from build123d import *

# Parameters (mm, degrees)
SKETCH1_R           = 0.6
BOSS_EXTRUDE1_DEPTH = 3
SKETCH1_22_R        = 0.9
SKETCH1_22_R_2      = 0.3
BOSS_EXTRUDE2_DEPTH = 8
SKETCH1_23_R        = 0.8
SKETCH1_23_R_2      = 0.3
BOSS_EXTRUDE3_DEPTH = 5


with BuildPart() as part:
    # Sketch1 → Boss-Extrude1 (new body)
    with BuildSketch(Plane(origin=(0, 0, 0), x_dir=(1, 0, 0), z_dir=(0, 1, 0))):
        with BuildLine():
            ThreePointArc((0.1641009, 1.993256355), (0.024548565, 1.994973575), (-0.113883759, 1.977245221))
            Line((-0.113883759, 1.977245221), (-4.183235691, 1.164159973))
            ThreePointArc((-4.183235691, 1.164159973), (-4.514100231, 1.033532975), (-4.77830642, 0.795352694))
            ThreePointArc((-4.77830642, 0.795352694), (-5.05, 0), (-4.77830642, -0.795352694))
            ThreePointArc((-4.77830642, -0.795352694), (-4.514100231, -1.033532975), (-4.183235691, -1.164159973))
            Line((-4.183235691, -1.164159973), (-0.11388376, -1.977245221))
            ThreePointArc((-0.11388376, -1.977245221), (0.024548564, -1.994973575), (0.164100898, -1.993256355))
            ThreePointArc((0.164100898, -1.993256355), (2, -1e-09), (0.1641009, 1.993256355))
        make_face()
        with Locations(Location((-1.25, 0, 0), (0, 0, 270))):
            Circle(SKETCH1_R, mode=Mode.SUBTRACT)
    extrude(amount=BOSS_EXTRUDE1_DEPTH)

    # Sketch1_22 → Boss-Extrude2 (add)
    # profile 1 of 2: a face of its own
    with BuildSketch(Plane(origin=(0, 0, 0), x_dir=(1, 0, 0), z_dir=(0, 1, 0))):
        with Locations(Location((0.5, 0, 0), (0, 0, 270))):
            Circle(SKETCH1_22_R)
        with Locations((0.5, 0)):
            Circle(SKETCH1_22_R_2, mode=Mode.SUBTRACT)
    # profile 2 of 2: a face of its own
    with BuildSketch(Plane(origin=(0, 0, 0), x_dir=(1, 0, 0), z_dir=(0, 1, 0))):
        with Locations((0.5, 0)):
            Circle(SKETCH1_22_R_2)
    extrude(amount=BOSS_EXTRUDE2_DEPTH)

    # Sketch1_23 → Boss-Extrude3 (add)
    # profile 1 of 2: a face of its own
    with BuildSketch(Plane(origin=(0, 0, 0), x_dir=(1, 0, 0), z_dir=(0, 1, 0))):
        with Locations(Location((-3, 0, 0), (0, 0, 270))):
            Circle(SKETCH1_23_R)
        with Locations((-3, 0)):
            Circle(SKETCH1_23_R_2, mode=Mode.SUBTRACT)
    # profile 2 of 2: a face of its own
    with BuildSketch(Plane(origin=(0, 0, 0), x_dir=(1, 0, 0), z_dir=(0, 1, 0))):
        with Locations((-3, 0)):
            Circle(SKETCH1_23_R_2)
    extrude(amount=BOSS_EXTRUDE3_DEPTH)


solid = part.part
Geometry check sheet. Reference: the model listing, model coordinates, mm. A direction names the side the tool comes from. Give positions to 0.01 mm unless a question says otherwise; leave off trailing zeros. Write each loop counter-clockwise with the first axis right and the second up, starting at its lowest first coordinate (ties: lowest second). Pieces come first, ordered by that corner, then holes. Notation, with made-up numbers: M 10.5,30.25 L 30.5,30.25 A14 ccw 30.5,41.25 Z; hole C -38,28.25 d1. An arc over 180 degrees is marked long. Answer as CSV lines item,"result". Start each with the question number.
Q1. Section check D-D, the plane z = -0.5. Record the cut outline in (x, y).
Q2. Section check C-C, the plane y = 5.5. Record the cut outline in (x, z).
Q3. Tool access check on faces 1 (the face through (-3.78, 3.99, -0.17)), 2 (the face through (-3, 5, 0)), 3 (the face through (-2, 0, 1)). Record the directions out of +Z, -Z, +X, -X, +Y, -Y that give a thin tool (end or side, any length) a straight path to the whole face; none if there is none.
Q4. Section check A-A, the plane z = 0. Record the cut outline in (x, y), then the cut area to 4 significant figures.
Q5. Material ranges on L1, parallel to X at y = 2.25, z = -0.35; L2, parallel to Y at x = -0.5, z = 1.1; L3, parallel to Z at x = 0.5, y = 7.25, recorded low to high.
Q6. Release check for a two-part mould opening along X. For faces 4 (the face through (1.39, 5.46, -0.12)), 5 (the face through (-2.12, 1.479, -1.576)), 6 (the face through (2, 1, 0)), 7 (the face through (1, 8, 0)) record: pulls with the +X half, pulls with the -X half, needs draft (parallel to the pull), parting line crosses it, or undercut.
Q7. Section check B-B, the plane x = -1.25. Record the cut outline in (y, z), then the cut area to 3 significant figures.
Q8. Go/stop test with flat-tipped pins: pin 1 (1.6 mm diameter, centred on x = -1.25, z = 0, fed in from +Y); pin 2 (1.3 mm diameter, centred on x = -3, z = 0.5, fed in from +Y); pin 3 (1 mm diameter, centred on x = -4, y = 4.5, fed in from +Z). Record where each tip stops, or that it passes through.
Geometry says:
1,outline,"M -4.95,0 L -1.58,0 L -1.58,3 L -2.38,3 L -2.38,5 L -3.62,5 L -3.62,3 L -4.95,3 Z; M -0.92,0 L 1.94,0 L 1.94,3 L 1.25,3 L 1.25,8 L -0.25,8 L -0.25,3 L -0.92,3 Z"
2,outline,"C 0.5,0 d1.8"
3,face 1,"+Y"
3,face 2,"+Z, -Z, -X, +Y"
3,face 3,"+Z, -Z, +X, -X, -Y"
4,outline,"M -5.05,0 L -1.85,0 L -1.85,3 L -2.2,3 L -2.2,5 L -3.8,5 L -3.8,3 L -5.05,3 Z; M -0.65,0 L 2,0 L 2,3 L 1.4,3 L 1.4,8 L -0.4,8 L -0.4,3 L -0.65,3 Z"
4,area,"29.75 mm^2"
5,L1,"-5 to -1.74, -0.76 to 1.97"
5,L2,"0 to 3"
5,L3,"-0.9 to 0.9"
6,face 4,"undercut"
6,face 5,"pulls with the -X half"
6,face 6,"pulls with the +X half"
6,face 7,"needs draft"
7,outline,"M 0,-1.75 L 3,-1.75 L 3,-0.6 L 0,-0.6 Z; M 0,0.6 L 3,0.6 L 3,1.75 L 0,1.75 Z"
7,area,"6.90 mm^2"
8,pin 1,"y = 3"
8,pin 2,"y = 5"
8,pin 3,"z = 0.62"
